Autodesk Inventor part; units mm, degrees
ref_plane "YZ Plane" through (0, 0, 0) normal (1, 0, 0) x (0, 1, 0)
ref_plane "XZ Plane" through (0, 0, 0) normal (0, 1, 0) x (-1, 0, 0)
ref_plane "XY Plane" through (0, 0, 0) normal (0, 0, 1) x (1, 0, 0)
ref_plane "Work Plane1" through (0, 0, 0) normal (0, 0, 1) x (1, 0, 0)
sketch "Sketch1" plane through (0, 0, 0) normal (0, 0, 1) x (1, 0, 0)
  circle A0 centre (11.5562, -18) radius 2 construction
  line L0 (-53.1938, -16) -> (-53.1938, -30) construction
  arc A1 (-56.1938, -30) -> (-53.1938, -30) centre (-54.6938, -30) ccw construction
  line L1 (-56.1938, -30) -> (-56.1938, -16) construction
  arc A2 (-53.1938, -16) -> (-56.1938, -16) centre (-54.6938, -16) ccw construction
  line L2 (7.0562, -16) -> (7.0562, -30) construction
  arc A3 (4.0562, -30) -> (7.0562, -30) centre (5.5562, -30) ccw construction
  line L3 (4.0562, -30) -> (4.0562, -16) construction
  arc A4 (7.0562, -16) -> (4.0562, -16) centre (5.5562, -16) ccw construction
  line L4 (-13.1938, -16) -> (-13.1938, -30) construction
  arc A5 (-16.1938, -30) -> (-13.1938, -30) centre (-14.6938, -30) ccw construction
  line L5 (-16.1938, -30) -> (-16.1938, -16) construction
  arc A6 (-13.1938, -16) -> (-16.1938, -16) centre (-14.6938, -16) ccw construction
  arc A7 (19.0562, -16) -> (16.0562, -16) centre (17.5562, -16) ccw construction
  line L6 (19.0562, -16) -> (19.0562, -30) construction
  arc A8 (16.0562, -30) -> (19.0562, -30) centre (17.5562, -30) ccw construction
  line L7 (16.0562, -30) -> (16.0562, -16) construction
  line L8 (22.8064, -40) -> (22.8064, 45) construction
  line L9 (22.8064, 45) -> (-120, 45) construction
  line L10 (-120, 27.5563) -> (-120, 45) construction
  line L11 (-120, 27.5563) -> (-95.2035, 27.5563) construction
  arc A9 (-85.0841, 27.5563) -> (-95.2035, 27.5563) centre (-90.1438, 25.4) ccw construction
  line L12 (-85.0841, 27.5563) -> (17.8062, 27.5563) construction
  line L13 (17.8062, 27.5563) -> (17.8062, -11) construction
  line L14 (17.8062, -11) -> (-120, -11) construction
  line L15 (-120, -40) -> (-120, -11) construction
  line L16 (22.8064, -40) -> (-120, -40) construction
  circle A10 centre (-111.1938, -18) radius 2 construction
  circle A11 centre (-98.1938, -18) radius 2 construction
  circle A12 centre (-61.1938, -18) radius 2 construction
  circle A13 centre (-48.1938, -18) radius 2 construction
  circle A14 centre (-21.1938, -18) radius 2 construction
  circle A15 centre (-8.1938, -18) radius 2 construction
  circle A16 centre (-21.1938, 33.6563) radius 2 construction
  circle A17 centre (-8.1938, 33.6563) radius 2 construction
  circle A18 centre (-61.1938, 33.6563) radius 2 construction
  circle A19 centre (-48.1938, 33.6563) radius 2 construction
  circle A20 centre (-111.1938, 33.6563) radius 2 construction
  circle A21 centre (-98.1938, 33.6563) radius 2 construction
  circle A22 centre (-90.1438, -25.4) radius 5.5 construction
  line L17 (5.3062, -11) -> (5.3062, 11) construction
  line L18 (17.8062, -11) -> (17.8062, 11) construction
  circle A23 centre (11.5562, 0) radius 3.75 construction
  line L19 (5.3062, -11) -> (17.8062, -11) construction
  arc A24 (-18.6938, -19.75) -> (-18.6938, -16.25) centre (-18.6938, -18) ccw construction
  line L20 (-18.6938, -16.25) -> (-23.6938, -16.25) construction
  arc A25 (-23.6938, -16.25) -> (-23.6938, -19.75) centre (-23.6938, -18) ccw construction
  line L21 (-23.6938, -19.75) -> (-18.6938, -19.75) construction
  arc A26 (-5.6938, -19.75) -> (-5.6938, -16.25) centre (-5.6938, -18) ccw construction
  line L22 (-5.6938, -16.25) -> (-10.6938, -16.25) construction
  arc A27 (-10.6938, -16.25) -> (-10.6938, -19.75) centre (-10.6938, -18) ccw construction
  line L23 (-10.6938, -19.75) -> (-5.6938, -19.75) construction
  line L24 (0.3062, -11) -> (0.3062, -25.3437) construction
  line L25 (0.3062, -25.3437) -> (-29.6938, -25.3437) construction
  line L26 (-29.6938, -11) -> (-29.6938, -25.3437) construction
  line L27 (0.3062, -11) -> (-29.6938, -11) construction
  line L28 (22.8064, -35.5) -> (0.3062, -35.5)
  line L29 (0.3062, -35.5) -> (0.3062, 0)
  line L30 (0.3062, 0) -> (7.7062, 0)
  line L31 (22.8064, 0) -> (22.8064, -35.5)
  arc A28 (7.7062, 0) -> (15.4062, 0) centre (11.5562, 0) ccw
  line L32 (11.5562, 15.4) -> (11.5562, -15.4) construction
  line L33 (-148.5613, 0) -> (51.3677, 0) construction
  line L34 (15.4062, 0) -> (22.8064, 0)
  point P0 (0, 0)
  point P1 (17.5562, -31.5)
  dimension "d0" = 0.1
  dimension "d1" = 0
  dimension "d2" = 0
  dimension "d3" = 4
extrude "Main Body" add sketch "Sketch1" along normal blind 5
sketch "Sketch2" plane through (0, 0, 0) normal (0, 0, -1) x (-1, 0, 0)
  line L0 (-16.0562, -30) -> (-16.0562, -16) construction
  arc A0 (-19.0562, -30) -> (-16.0562, -30) centre (-17.5562, -30) ccw construction
  line L1 (-19.0562, -16) -> (-19.0562, -30) construction
  arc A1 (-16.0562, -16) -> (-19.0562, -16) centre (-17.5562, -16) ccw construction
  arc A2 (-7.0562, -30) -> (-4.0562, -30) centre (-5.5562, -30) ccw construction
  line L2 (-7.0562, -16) -> (-7.0562, -30) construction
  arc A3 (-4.0562, -16) -> (-7.0562, -16) centre (-5.5562, -16) ccw construction
  line L3 (-4.0562, -30) -> (-4.0562, -16) construction
  line L4 (-17.5562, -30) -> (-17.5562, -16) construction
  line L5 (-5.5562, -16) -> (-5.5562, -30) construction
  line L6 (-17.5562, -29) -> (-17.5562, -17) construction
  line L7 (-16.1062, -29) -> (-16.1062, -17)
  line L8 (-19.0062, -17) -> (-19.0062, -29)
  arc A4 (-19.0062, -29) -> (-16.1062, -29) centre (-17.5562, -29) ccw
  arc A5 (-16.1062, -17) -> (-19.0062, -17) centre (-17.5562, -17) ccw
  line L9 (-5.5562, -29) -> (-5.5562, -17) construction
  line L10 (-4.1062, -29) -> (-4.1062, -17)
  line L11 (-7.0062, -17) -> (-7.0062, -29)
  arc A6 (-7.0062, -29) -> (-4.1062, -29) centre (-5.5562, -29) ccw
  arc A7 (-4.1062, -17) -> (-7.0062, -17) centre (-5.5562, -17) ccw
  line L12 (-17.5562, -29) -> (-5.5562, -29) construction
  line L13 (-17.5562, -17) -> (-5.5562, -17) construction
  point P0 (0, 0)
  point P1 (-17.5562, -23)
  point P2 (-5.5562, -23)
  dimension "d6" = 1
  dimension "d7" = 0.05
  dimension "d8" = 0.05
extrude "Alignment Tabs" add sketch "Sketch2" along normal blind 1.8
sketch "Sketch3" plane through (0, 0, 5) normal (0, 0, 1) x (1, 0, 0)
  circle A0 centre (11.5562, -18) radius 2 construction
  line L0 (11.5562, -19.5) -> (11.5562, -16.5) construction
  line L1 (13.3062, -19.5) -> (13.3062, -16.5)
  line L2 (9.8062, -16.5) -> (9.8062, -19.5)
  arc A1 (9.8062, -19.5) -> (13.3062, -19.5) centre (11.5562, -19.5) ccw
  arc A2 (13.3062, -16.5) -> (9.8062, -16.5) centre (11.5562, -16.5) ccw
  point P0 (0, 0)
  dimension "d11" = 3.5
  dimension "d12" = 3
extrude "Slot for Screw M3" cut sketch "Sketch3" against normal through all
equation "\"d8\" = d7"
properties part number "Cuvette Aligner 10mm"
Geometry check sheet. Reference: the model listing, model coordinates, mm. A direction names the side the tool comes from. Give positions to 0.01 mm unless a question says otherwise; leave off trailing zeros. Order: outer loops, then holes, each group sorted by start corner. A loop starts at its lowest first (then second) coordinate and runs counter-clockwise, first axis right, second up. Notation, with made-up numbers: (-39.5, 17.5) -> (6.5, 17.5) arc R24 cw to (6.5, 52.5) -> close; hole circle Ø5 at (-29.5, -13.75). An arc over 180 degrees is marked (long way). Write each question's results on one line, items separated by ' | '. Start each with the question number.
(1) Sectioned sample at C-C (x = 3). Enter the section's corners in (y, z).
(2) Sectioned sample at A-A (z = 3.5). Enter the section's corners in (x, y).
(3) Access from +Z, -Z, +X, -X, +Y, -Y to the whole of each face (thin tool, end or side, straight path). Record for faces 1 (the face through (17.52, -30.45, -0.89)), 2 (the face through (11.59, -14.75, 2.54)), 3 (the face through (19.006, -23, -1)).
(4) Gauge pin test, flat ends, axial feed: P1, Ø1.5, axis at x = 3, y = -24, coming from the -Z side; P2, Ø2, axis at y = -22, z = -0.5, coming from the +X side; P3, Ø0.5, axis at y = -23, z = -1, coming from the +X side. Record the tip position at first contact, or that the pin passes through.
(5) Sectioned sample at B-B (y = -23). Enter the section's corners in (x, z), plus the area to 3 significant figures.
(6) Mould release check, pull along X, two halves, no side actions. Record for faces 4 (the face through (11.64, -3.85, 2.46)), 5 (the face through (4.106, -23, -1)), 6 (the face through (6, -23, -1.8)): pulls with the +X half, pulls with the -X half, needs draft (parallel to the pull), parting line crosses it, or undercut.
(7) Sectioned sample at D-D (y = -31.5). Enter the section's corners in (x, z), plus the area to 3 significant figures.
(8) Scan lines: line 1 (X direction, y = -25, z = -1.5); line 2 (Z direction, x = 18.25, y = -9); line 3 (X direction, y = -16.5, z = 2.25). Record each from-to range of solid material in increasing order.
Answer below:
1) outline: (-35.5, 0) -> (0, 0) -> (0, 5) -> (-35.5, 5) -> close
2) outline: (0.31, -35.5) -> (22.81, -35.5) -> (22.81, 0) -> (15.41, 0) arc R3.85 cw to (7.71, 0) -> (0.31, 0) -> close; hole (9.81, -19.5) arc R1.75 ccw to (13.31, -19.5) -> (13.31, -16.5) arc R1.75 ccw to (9.81, -16.5) -> close
3) face 1: -Z, -Y | face 2: +Z, -Z | face 3: -Z, +X, +Y, -Y
4) P1: z = 0 | P2: x = 22.81 | P3: x = 19.01
5) outline: (0.31, 0) -> (4.11, 0) -> (4.11, -1.8) -> (7.01, -1.8) -> (7.01, 0) -> (16.11, 0) -> (16.11, -1.8) -> (19.01, -1.8) -> (19.01, 0) -> (22.81, 0) -> (22.81, 5) -> (0.31, 5) -> close | area: 123 mm2
6) face 4: undercut | face 5: pulls with the -X half | face 6: needs draft
7) outline: (0.31, 0) -> (22.81, 0) -> (22.81, 5) -> (0.31, 5) -> close | area: 113 mm2
8) line 1: 4.11 to 7.01, 16.11 to 19.01 | line 2: 0 to 5 | line 3: 0.31 to 9.81, 13.31 to 22.81
